Can you work these out from the model? Positions are in its coordinate system, mm. A direction names the side the tool comes from. Coordinates: 2 decimals unless noted, no trailing zeros. Loops run counter-clockwise (first coordinate to the right, second up) from the corner with the lowest first, then second, coordinate; pieces in that order, holes last. Notation, with made-up numbers: (85, -36.5) -> (126, -36.5) arc R18 ccw to (126, -21.5) -> close; hole circle Ø5 at (-18.5, 84.25). An arc over 180 degrees is marked (long way). Put each result on its own line as item: value. Start each with the question number.
Item 1: If we section it at B-B on z = 7: Please give me the cut outline in (x, y) (3 decimals).
Item 2: If we section it at C-C on x = 17.5: Please give me the cut outline in (y, z).
Item 3: Will these pins go through, and if not, where does the flat tip stop? P1, Ø4, axis at x = 20.39, y = -9.51, coming from the +Z side; P2, Ø2, axis at y = 3, z = 23.5, coming from the -X side; P3, Ø6, axis at y = -20.5, z = 17.5, coming from the -X side.
Item 4: For faces 1 (the flat face through (5.5, -20, 14)), 2 (the cylindrical face through (15.69, 11.12, 16.05)), 3 (the cylindrical face through (3.15, -25.1, 19.86)), 4 (the flat face through (2.5, -20, 14)), which set-ups out of +Z, -Z, +X, -X, +Y, -Y let a thin tool reach every point of the face, with its end or its side?
Item 5: If we section it at D-D on y = 13.5: Please give me the cut outline in (x, z), plus the area to 3 significant figures.
Item 6: Please list where these lines run through material, in increasing order: L1, parallel to Z at x = 22.5, y = 3.5; L2, parallel to X at y = -20, z = 15; L3, parallel to X at y = 10.5, z = 27. Write a range as from..to.
Item 7: If we section it at A-A on y = 0: Please give me the cut outline in (x, z), plus the area to 3 significant figures.
Item 8: We'd pull the mould along Y, two halves only. Please class faces 5 (the flat face through (17.92, -13.68, 0.18)), 6 (the flat face through (17.6, 5.6, 30)), 7 (the cylindrical face through (20.921, 0.496, 0.179)), 8 (the cylindrical face through (1.79, -23.08, 4.27)): pulls with the +Y half, pulls with the -Y half, needs draft (parallel to the pull), parting line crosses it, or undercut.
```python
from build123d import *

# Parameters (mm, degrees)
EXTRUDE_1_DEPTH     = 31.3
EXTRUDE_2_DEPTH     = 3
EXTRUDE_3_DEPTH     = 31.3
SKETCH_9_W          = 7.730582044
SKETCH_9_H          = 5.996077833
CUT_EXTRUDE_1_DEPTH = 20
ST2_9_1_D           = 3.3
FILLET_1_R          = 1
FILLET_2_R          = 2


with BuildPart() as part:
    # 草图1 → 凸台-拉伸1 (new body)
    with BuildSketch(Plane.XY.offset(-1.3)):
        with BuildLine():
            Line((36.062445841, 36.062445841), (11.313708499, 11.313708499))
            ThreePointArc((11.313708499, 11.313708499), (15.216442494, -4.945692856), (2.5, -15.803480629))
            Line((2.5, -15.803480629), (2.5, -18.834808202))
            ThreePointArc((2.5, -18.834808202), (17.455469833, -7.50377058), (15.387819505, 11.145178818))
            Line((15.387819505, 11.145178818), (38.183766184, 33.941125497))
            Line((38.183766184, 33.941125497), (36.062445841, 36.062445841))
        make_face()
    extrude(amount=EXTRUDE_1_DEPTH)

    # 草图2 → 凸台-拉伸2 (add)
    with BuildSketch(Plane.XY.offset(-1.3)):
        with BuildLine():
            Line((15.387819505, 11.145178818), (20.383302711, 16.140662024))
            ThreePointArc((20.383302711, 16.140662024), (26, 0), (20.383302711, -16.140662024))
            Line((20.383302711, -16.140662024), (15.387819505, -11.145178818))
            ThreePointArc((15.387819505, -11.145178818), (19, 0), (15.387819505, 11.145178818))
        make_face()
    extrude(amount=EXTRUDE_2_DEPTH)

    # 草图8 → 凸台-拉伸3 (add)
    with BuildSketch(Plane.XY.offset(-1.3)):
        with BuildLine():
            Line((2.5, -18.834808202), (2.5, -21.334808202))
            ThreePointArc((2.5, -21.334808202), (1.767766953, -23.102575155), (0, -23.834808202))
            Line((0, -23.834808202), (0, -26.834808202))
            ThreePointArc((0, -26.834808202), (3.889087297, -25.223895498), (5.5, -21.334808202))
            Line((5.5, -21.334808202), (5.5, -18.186533479))
            ThreePointArc((5.5, -18.186533479), (4.013111639, -18.57134715), (2.5, -18.834808202))
        make_face()
    extrude(amount=EXTRUDE_3_DEPTH)

    # 草图9 → 切除-拉伸1 (cut)
    with BuildSketch(Plane.XY.offset(30)):
        with Locations((-1.365291022, -24.332847119)):
            Rectangle(SKETCH_9_W, SKETCH_9_H)
    extrude(amount=-CUT_EXTRUDE_1_DEPTH, mode=Mode.SUBTRACT)

    # ST2.9 间隙孔1 (through all)
    with Locations(Plane.XY.offset(1.7)):
        with Locations((22.494945516, 0), (20.38734429, 9.506774772), (20.38734429, -9.506774772)):
            Hole(ST2_9_1_D / 2)

    # 圆角1
    fillet_1_edges = [part.edges().sort_by_distance(p)[0] for p in [
        (2.5, -15.803480629, 14.35),
        (15.387819505, 11.145178818, 15.85),
        (5.5, -18.186533479, 14.35),
        (2.5, -26.233787687, 20),
    ]]
    fillet(fillet_1_edges, radius=FILLET_1_R)

    # 圆角2
    fillet_2_edges = [part.edges().sort_by_distance(p)[0] for p in [
        (11.313708499, 11.313708499, 14.35),
    ]]
    fillet(fillet_2_edges, radius=FILLET_2_R)


solid = part.part
```
Solutions:
1. outline: (0, -26.835) arc R5.5 ccw to (5.5, -21.335) -> (5.5, -18.914) arc R1 cw to (6.175, -17.969) arc R19 ccw to (15.851, 10.477) arc R1 cw to (15.978, 11.735) -> (38.184, 33.941) -> (36.062, 36.062) -> (12.649, 12.649) arc R2 ccw to (12.501, 9.987) arc R16 cw to (3.294, -15.657) arc R1 ccw to (2.5, -16.636) -> (2.5, -21.335) arc R2.5 cw to (0, -23.835) -> close
2. outline: (-13.26, -1.3) -> (17.5, -1.3) -> (17.5, 30) -> (13.26, 30) -> (13.26, 1.7) -> (7.4, 1.7) -> (7.4, 30) -> (-7.4, 30) -> (-7.4, 1.7) -> (-13.26, 1.7) -> close
3. P1: z = 1.7
3. P2: x = 15.49
3. P3: x = 2.5
4. face 1: +Z, -Z, +X, -Y
4. face 2: +Z, +X
4. face 3: +Z, -Y
4. face 4: +Z, -X, +Y
5. outline: (13.5, -1.3) -> (22.22, -1.3) -> (22.22, 1.7) -> (17.74, 1.7) -> (17.74, 30) -> (13.5, 30) -> close
5. area: 146 mm^2
6. L1: -1.3..1.7
6. L2: 2.5..5.5
6. L3: 12.2..15.84
7. outline: (16, -1.3) -> (20.84, -1.3) -> (20.84, 1.7) -> (19, 1.7) -> (19, 30) -> (16, 30) -> close; (24.14, -1.3) -> (26, -1.3) -> (26, 1.7) -> (24.14, 1.7) -> close
7. area: 105 mm^2
8. face 5: pulls with the -Y half
8. face 6: needs draft
8. face 7: undercut
8. face 8: pulls with the +Y half
